```python
from build123d import *

# Parameters (mm, degrees)
SKETCH_1_R          = 18.5
EXTRUDE_1_DEPTH     = 25
SKETCH_3_R          = 13.75
EXTRUDE_2_DEPTH     = 40
SKETCH_4_R          = 1.5
CUT_EXTRUDE_1_DEPTH = 3
SKETCH_5_R          = 6
EXTRUDE_3_DEPTH     = 6
SKETCH_6_R          = 3
EXTRUDE_4_DEPTH     = 15
CUT_EXTRUDE_2_DEPTH = 12
SKETCH_8_R          = 5.1
EXTRUDE_5_DEPTH     = 3


with BuildPart() as part:
    # ｽｹｯﾁ1 → ﾎﾞｽ - 押し出し1 (new body)
    with BuildSketch(Plane.XY):
        Circle(SKETCH_1_R)
    extrude(amount=EXTRUDE_1_DEPTH)

    # ｽｹｯﾁ3 → ﾎﾞｽ - 押し出し2 (add)
    with BuildSketch(Plane.XY.offset(25)):
        Circle(SKETCH_3_R)
    extrude(amount=EXTRUDE_2_DEPTH)

    # ｽｹｯﾁ4 → ｶｯﾄ - 押し出し1 (cut)
    with BuildSketch(Plane(origin=(0, 0, 0), x_dir=(-1, 0, 0), z_dir=(0, 0, -1))):
        with Locations((-7.75, 13.423393759)):
            Circle(SKETCH_4_R)
        with Locations((-7.75, -13.423393759)):
            Circle(SKETCH_4_R)
        with Locations((15.5, 0)):
            Circle(SKETCH_4_R)
    extrude(amount=-CUT_EXTRUDE_1_DEPTH, mode=Mode.SUBTRACT)

    # ｽｹｯﾁ5 → ﾎﾞｽ - 押し出し3 (add)
    with BuildSketch(Plane(origin=(0, 0, 0), x_dir=(-1, 0, 0), z_dir=(0, 0, -1))):
        with Locations((0, -7)):
            Circle(SKETCH_5_R)
    extrude(amount=EXTRUDE_3_DEPTH)

    # ｽｹｯﾁ6 → ﾎﾞｽ - 押し出し4 (add)
    with BuildSketch(Plane(origin=(0, 0, -6), x_dir=(-1, 0, 0), z_dir=(0, 0, -1))):
        with Locations((0, -7)):
            Circle(SKETCH_6_R)
    extrude(amount=EXTRUDE_4_DEPTH)

    # ｽｹｯﾁ7 → ｶｯﾄ - 押し出し2 (cut)
    with BuildSketch(Plane(origin=(0, 0, -21), x_dir=(-1, 0, 0), z_dir=(0, 0, -1))):
        with BuildLine():
            ThreePointArc((1.658312395, -4.5), (0, -4), (-1.658312395, -4.5))
            Line((-1.658312395, -4.5), (1.658312395, -4.5))
        make_face()
    extrude(amount=-CUT_EXTRUDE_2_DEPTH, mode=Mode.SUBTRACT)

    # ｽｹｯﾁ8 → ﾎﾞｽ - 押し出し5 (add)
    with BuildSketch(Plane.XY.offset(65)):
        Circle(SKETCH_8_R)
    extrude(amount=EXTRUDE_5_DEPTH)


solid = part.part
```
For this review, take the finished solid that the model builds, in its own axes (mm). A direction names the side the tool comes from. Give positions to 0.01 mm unless a question says otherwise; leave off trailing zeros. Write each loop counter-clockwise with the first axis right and the second up, starting at its lowest first coordinate (ties: lowest second). Pieces come first, ordered by that corner, then holes. Notation, with made-up numbers: M -24.75,88.5 L 12.25,88.5 A9 ccw 12.25,97.5 Z; hole C 65,-5.75 d8. An arc over 180 degrees is marked long. One line per item, written item: value.
1) Take a section at A-A, the plane x = 0. Write out the cut boundary in (y, z), then the cut area to 3 significant figures.
Results are:
outline: M -18.5,0 L -13,0 L -13,-6 L -10,-6 L -10,-21 L -4.5,-21 L -4.5,-9 L -4,-9 L -4,-6 L -1,-6 L -1,0 L 18.5,0 L 18.5,25 L 13.75,25 L 13.75,65 L 5.1,65 L 5.1,68 L -5.1,68 L -5.1,65 L -13.75,65 L -13.75,25 L -18.5,25 Z
area: 2,210 mm²
2) Take a section at B-B, the plane y = 0. Write out the cut boundary in (x, z).
Results are:
outline: M -18.5,0 L -17,0 L -17,3 L -14,3 L -14,0 L 18.5,0 L 18.5,25 L 13.75,25 L 13.75,65 L 5.1,65 L 5.1,68 L -5.1,68 L -5.1,65 L -13.75,65 L -13.75,25 L -18.5,25 Z
3) The part is to be moulded in two halves that separate along X. For faces 5 (the cylindrical face through (-2.981, -13.423, 44.72)), 6 (the flat face through (8, -13, 3)), 7 (the flat face through (3, -8, -6)), say which applies: +X half, -X half, draft (parallel to the pull), parting line (faces both ways), or undercut.
Results are:
face 5: parting line
face 6: undercut
face 7: draft
4) For faces 1 (the flat face through (0, 14, 25)), 2 (the cylindrical face through (6, -7, -3)), 3 (the cylindrical face through (-4.01, -18.06, 12.32)), 4 (the flat face through (0, -4.5, -15)), list the 3-axis set-ups (+Z, -Z, +X, -X, +Y, -Y) from which the entire face can be reached by the end or side of a thin tool; tool diameter is ignored.
Results are:
face 1: +Z
face 2: -Z
face 3: +Z, -Z
face 4: -Z, +X, -X, +Y
5) Take a section at C-C, the plane z = -10.5. Write out the cut boundary in (x, y).
Results are:
outline: M -1.66,-4.5 A3 ccw long 1.66,-4.5 Z
6) Take a section at D-D, the plane y = 10. Write out the cut boundary in (x, z).
Results are:
outline: M -15.56,0 L 15.56,0 L 15.56,25 L 9.44,25 L 9.44,65 L -9.44,65 L -9.44,25 L -15.56,25 Z
7) For P1, Ø3.5, axis at x = 8, y = -13, coming from the -Z side; P2, Ø6, axis at x = -2, y = 10, coming from the +Z side; P3, Ø8, axis at x = -7.5, z = -4.5, coming from the +Y side; P4, Ø11, axis at x = -5, y = -4.5, coming from the +Z side, all flat-tipped, find the tip position at first contact; note any pin that passes through.
Results are:
P1: stops at z = 0
P2: stops at z = 65
P3: stops at y = -2.13
P4: stops at z = 68
8) For line 1 (Y direction, x = 7.75, z = 0.85); line 2 (Z direction, x = 4, y = 15.5); line 3 (Z direction, x = -2, y = -12), list the stretches that pass through material, from the lowest coordinate up. Write a range as from..to.
Results are:
line 1: y = -16.8..-14.92, -11.92..11.92, 14.92..16.8
line 2: z = 0..25
line 3: z = -6..65
